Autodesk Inventor part; units mm, degrees
ref_plane "YZ Plane" through (0, 0, 0) normal (1, 0, 0) x (0, 1, 0)
ref_plane "XZ Plane" through (0, 0, 0) normal (0, 1, 0) x (-1, 0, 0)
ref_plane "XY Plane" through (0, 0, 0) normal (0, 0, 1) x (1, 0, 0)
sketch "Sketch1" plane through (0, 0, 0) normal (0, 0, 1) x (1, 0, 0)
  line L0 (0, 0) -> (-133.543, 0)
  line L1 (-133.543, 0) -> (-133.543, -1490)
  line L2 (-133.543, -1490) -> (0, -1490)
  line L3 (0, -1490) -> (0, 0)
  line L4 (-133.543, -1390) -> (-66, -1390)
  line L5 (-66, -1390) -> (-66, -1385)
  line L6 (-66, -1385) -> (-133.543, -1385)
  line L7 (-133.543, -1385) -> (-133.543, -1390)
  line L8 (-133.543, -893.3333) -> (-66, -893.3333)
  line L9 (-66, -893.3333) -> (-66, -888.3333)
  line L10 (-66, -888.3333) -> (-133.543, -888.3333)
  line L11 (-133.543, -888.3333) -> (-133.543, -893.3333)
  line L12 (-133.543, -396.6667) -> (-66, -396.6667)
  line L13 (-66, -396.6667) -> (-66, -391.6667)
  line L14 (-66, -391.6667) -> (-133.543, -391.6667)
  line L15 (-133.543, -391.6667) -> (-133.543, -396.6667)
  circle A0 centre (-133.543, -155) radius 30
  point P0 (-133.543, -391.6667)
  point P1 (-133.543, -125)
  point P2 (-133.543, -185)
  dimension "d0" = 1490
  dimension "d1" = 133.543
  dimension "d2" = 5
  dimension "d4" = 100
  dimension "d7" = 496.6667
  dimension "d23" = 66
  dimension "d28" = 60
  dimension "d29" = 1335
extrude "Plate1" add sketch "Sketch1" along normal blind 4 contours L3 L2 L1 L4 L5 L6 L8 L9 L10 L12 L13 L14 A0 L0
sketch "Sketch2" plane through (4, 0, 0) normal (-1, 0, 0) x (0, -1, 0)
  line L0 (1490, 0) -> (0, 0)
  line L1 (0, 0) -> (0, 60)
  line L2 (0, 60) -> (1490, 60)
  line L3 (1490, 60) -> (1490, 0)
edge flange "Flange1" height 60 angle 90 thickness 4 bend radius 4 thickness toward (-1, 0, 0) relief tear relief width 4 relief depth 2 edges at (0, -745, 4) wall of the first edge with corners at (4, -1490, 0) (4, 0, 0) (4, 0, 60) (4, -1490, 60)
bend "Bend1"
corner "Corner1"
chamfer "Corner Chamfer1" distance 3 angle 45 6 edges at (-133.543, -1390, 2) (-133.543, -1385, 2) (-133.543, -893.3333, 2) (-133.543, -888.3333, 2) (-133.543, -391.6667, 2) (-133.543, -396.6667, 2)
equation "\"d0\" = Стрингер_длина"
equation "\"d1\" = стрингер_глубина_6"
equation "\"d2\" = паз_под_стрингер_толщина"
equation "\"d7\" = 0.333333 * Стрингер_длина"
equation "\"d23\" = паз_под_стрингер_глубина - Thickness"
equation "\"d28\" = 2 * радиус_выреза_под_сварку"
equation "\"d12\" = Thickness"
equation "\"d13\" = BendReliefWidth"
equation "\"d14\" = BendReliefDepth"
equation "\"d15\" = MinimumRemnant"
equation "\"d16\" = TransitionRadius"
equation "\"d17\" = ребро_усилителей"
equation "\"d19\" = BendRadius"
equation "\"d20\" = CornerReliefSize"
equation "\"d21\" = GapSize"
equation "\"d22\" = JacobiRadiusSize"
equation "\"BendRadius\" = Thickness"
equation "\"BendReliefWidth\" = Thickness"
equation "\"BendReliefDepth\" = 0.5 * Thickness"
equation "\"CornerReliefSize\" = 4 * Thickness"
equation "\"MinimumRemnant\" = 2 * Thickness"
equation "\"TransitionRadius\" = BendRadius"
equation "\"JacobiRadiusSize\" = BendRadius"
equation "\"GapSize\" = Thickness"
properties part number "GBK 1214 stringer 6" material "Steel"
Here's how the part is built. I have some questions about the finished solid (model axes, mm). A direction names the side the tool comes from. Coordinates: 2 decimals unless noted, no trailing zeros. Write each loop counter-clockwise with the first axis right and the second up, starting at its lowest first coordinate (ties: lowest second). Pieces come first, ordered by that corner, then holes.
Item 1: If we mould it in two halves opening along Y, with no side actions, what happens to faces 1 (the flat face through (4, -735, 34)), 2 (the flat face through (-44, -1490, 3)), 3 (the cylindrical face through (-103.55, -154.34, 1.97))? For each: +Y half, -Y half, draft (parallel to the pull), parting line (faces both ways), or undercut.
Item 2: Will these pins go through, and if not, where does the flat tip stop? pin 1 (1.2 mm diameter, centred on y = -1387.5, z = 2.5, fed in from -X); pin 2 (3 mm diameter, centred on y = -506.5, z = 19.5, fed in from -X); pin 3 (4.5 mm diameter, centred on y = -393.5, z = 2.5, fed in from -X).
Item 3: I want a section at D-D on x = -16.5. Write out the boundary of the cut face in (y, z), and give its area (3 significant figures).
Item 4: I want a section at A-A on y = -1248.5. Write out the boundary of the cut face in (x, z), and give its area (3 significant figures).
Item 5: On a 3-axis mill with a long thin cutter (end or side, diameter ignored), from which of +Z, -Z, +X, -X, +Y, -Y can I reach the whole of each face in a straight line? I mean faces 4 (the flat face through (-44, 0, 3)), 5 (the flat face through (0, -735, 34)). Say none if no direction works.
Item 6: I want a section at C-C on z = 25.5. Write out the boundary of the cut face in (x, y), and give its area (3 significant figures).
Item 7: I want a section at B-B on y = -155. Write out the boundary of the cut face in (x, z).
Item 8: If I drill on line 1 (Z direction, x = -57, y = -625.5); line 2 (X direction, y = -654.5, z = 6.5), over which ranges is the centre line in solid material (lowest first)?
Findings below:
1. face 1: draft
1. face 2: -Y half
1. face 3: undercut
2. pin 1: stops at x = -66
2. pin 2: stops at x = 0
2. pin 3: stops at x = -130.96
3. outline: (-1490, 0) - (0, 0) - (0, 4) - (-1490, 4) - close
3. area: 5,960 mm2
4. outline: (-133.54, 0) - (-4, 0) arc R8 ccw to (4, 8) - (4, 60) - (0, 60) - (0, 8) arc R4 cw to (-4, 4) - (-133.54, 4) - close
4. area: 764 mm2
5. face 4: +Z, -Z, +X, -X, +Y
5. face 5: +Z, -X, +Y, -Y
6. outline: (0, -1490) - (4, -1490) - (4, 0) - (0, 0) - close
6. area: 5,960 mm2
7. outline: (-103.54, 0) - (-4, 0) arc R8 ccw to (4, 8) - (4, 60) - (0, 60) - (0, 8) arc R4 cw to (-4, 4) - (-103.54, 4) - close
8. line 1: z = 0 to 4
8. line 2: x = -0.29 to 3.86
